Geometry check sheet. Reference: drawing and pictorial views, mm from the part's lowest x, y, z. A direction names the side the tool comes from. Give positions to 0.01 mm unless a question says otherwise; leave off trailing zeros. Order: outer loops, then holes, each group sorted by start corner. A loop starts at its lowest first (then second) coordinate and runs counter-clockwise, first axis right, second up.
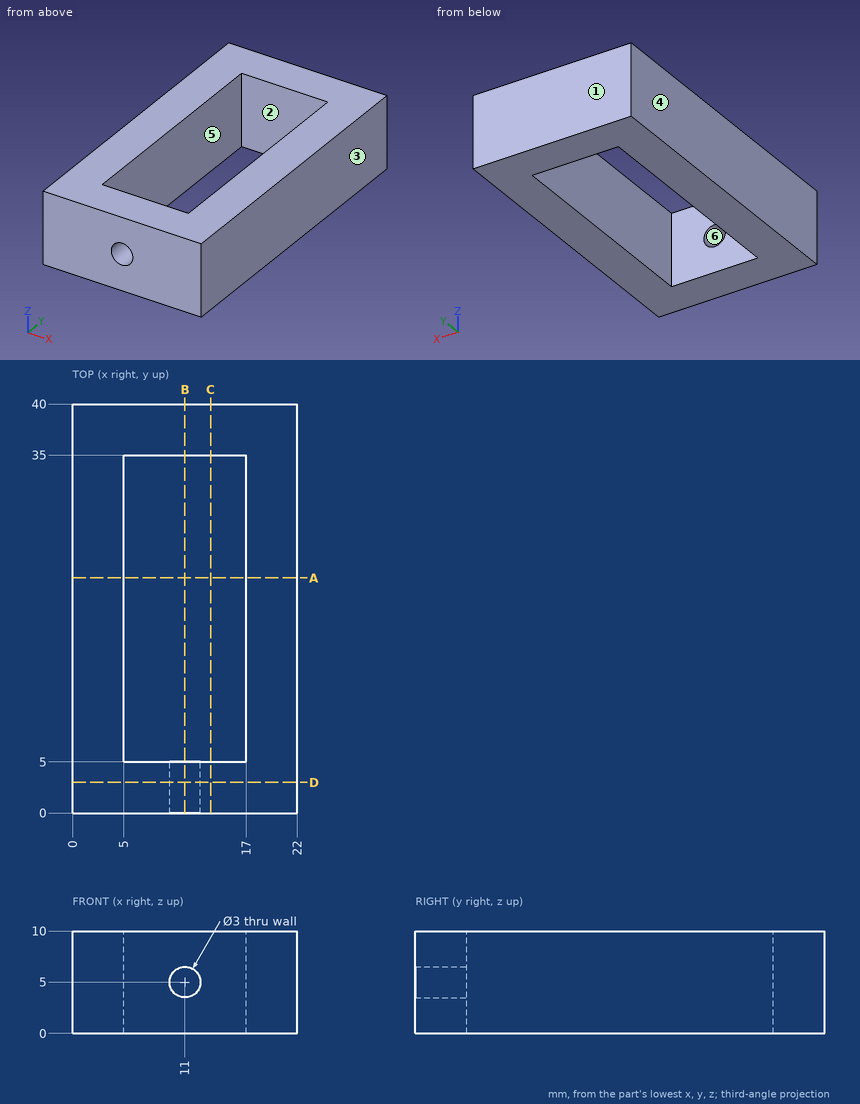
1) Section check D-D, the plane y = 3. Record the cut outline in (x, z).
Recorded:
outline: (0, 0) - (22, 0) - (22, 10) - (0, 10) - close; hole circle Ø3 at (11, 5)
2) Section check C-C, the plane x = 13.5. Record the cut outline in (y, z).
Recorded:
outline: (0, 0) - (5, 0) - (5, 10) - (0, 10) - close; (35, 0) - (40, 0) - (40, 10) - (35, 10) - close
3) Draft check along X on the marked faces 1, 2 and 3. Enter one of: +X half, -X half, draft (parallel to the pull), parting line (faces both ways), or undercut.
Recorded:
face 1: draft
face 2: undercut
face 3: +X half
4) Section check B-B, the plane x = 11. Record the cut outline in (y, z).
Recorded:
outline: (0, 0) - (5, 0) - (5, 3.5) - (0, 3.5) - close; (0, 6.5) - (5, 6.5) - (5, 10) - (0, 10) - close; (35, 0) - (40, 0) - (40, 10) - (35, 10) - close
5) Material ranges on L1, parallel to X at y = 2.7, z = 5; L2, parallel to X at y = 20, z = 6.25; L3, parallel to Y at x = 16, z = 3.75, recorded low to high.
Recorded:
L1: x = 0 to 9.5, 12.5 to 22
L2: x = 0 to 5, 17 to 22
L3: y = 0 to 5, 35 to 40
6) Set-up check for the marked faces 4, 5 and 6: record each of +Z, -Z, +X, -X, +Y, -Y from which the full face is reachable in a straight line by a thin tool's end or side.
Recorded:
face 4: +Z, -Z, -X, +Y, -Y
face 5: +Z, -Z
face 6: -Y
7) Section check A-A, the plane y = 23. Record the cut outline in (x, z), then the cut area to 3 significant figures.
Recorded:
outline: (0, 0) - (5, 0) - (5, 10) - (0, 10) - close; (17, 0) - (22, 0) - (22, 10) - (17, 10) - close
area: 100 mm2
